Can you work these out from the model? Positions are in its coordinate system, mm. A direction names the side the tool comes from. Round coordinates to 2 decimals unless told otherwise and drop trailing zeros. Write each loop counter-clockwise with the first axis right and the second up, starting at its lowest first coordinate (ties: lowest second). Pieces come first, ordered by that corner, then holes.
Q1. We'd pull the mould along Y, two halves only. Please class faces 1 (the flat face through (9.75, 0, 1)), 2 (the flat face through (-11.5, 0, 1)), 3 (the flat face through (-10, 42, 1)), 4 (the flat face through (-7.5, -43, 1)): +Y half, -Y half, draft (parallel to the pull), parting line (faces both ways), or undercut.
Q2. If we section it at C-C (z = 0.9): Give the number of separate pieces and of enclosed holes in the cut face, plus the area to 3 significant figures.
Q3. If we section it at A-A (x = 0): Please give me the cut outline in (y, z), plus the area to 3 significant figures.
Q4. For faces 5 (the flat face through (7.5, 43, 1)), 6 (the flat face through (5.25, 0, 1)), 7 (the flat face through (-7.5, 43, 1)), 8 (the flat face through (2, -42, 1)), which set-ups out of +Z, -Z, +X, -X, +Y, -Y let a thin tool reach every point of the face, with its end or its side?
Q5. If we section it at D-D (x = -5.5): Please give me the cut outline in (y, z).
Q6. If we section it at B-B (y = -27): Please give me the cut outline in (x, z), plus the area to 3 significant figures.
Q7. Please list where these lines run through material, in increasing order: line 1 along Y through (x, z) = (-8.65, 0.95); line 2 along Y through (x, z) = (0.5, 1.8); line 3 along Y through (x, z) = (-10.75, 1.6).
Q8. I'm going to push flat-ended pins straight in: pin 1 Ø0.9 at (y, z) = (43.5, 1.5) entering from -X; pin 2 Ø0.9 at (y, z) = (-29, 1) entering from -X; pin 3 Ø1.6 at (x, z) = (-11, 1) entering from -Y; pin 4 Ø1.2 at (x, y) = (-8.65, -21.175) entering from -Z. Where does each tip first touch, or does it pass through?
from build123d import *

# Parameters (mm, degrees)
CROQUIS2_W              = 25
CROQUIS2_H              = 90
SALIENTE_EXTRUIR1_DEPTH = 3
CROQUIS3_W              = 10
CROQUIS3_H              = 3
CROQUIS3_W_2            = 5
CORTAR_EXTRUIR1_DEPTH   = 47.800106837
CROQUIS5_R              = 8.5
CROQUIS5_R_2            = 0.975
CORTAR_EXTRUIR2_DEPTH   = 47.800106837
CROQUIS6_W              = 2
CROQUIS6_H              = 11
CORTAR_EXTRUIR3_DEPTH   = 10
CROQUIS7_W              = 3
CROQUIS7_H              = 25
SALIENTE_EXTRUIR2_DEPTH = 3
CHAFL_N1_SIZE           = 3


with BuildPart() as part:
    # Croquis2 → Saliente-Extruir1 (new body)
    with BuildSketch(Plane.XY):
        Rectangle(CROQUIS2_W, CROQUIS2_H)
    extrude(amount=SALIENTE_EXTRUIR1_DEPTH)

    # Croquis3 → Cortar-Extruir1 (cut, through all)
    with BuildSketch(Plane.XY):
        with Locations((2.5, 43.5)):
            Rectangle(CROQUIS3_W, CROQUIS3_H)
        with Locations((-10, 43.5)):
            Rectangle(CROQUIS3_W_2, CROQUIS3_H)
    cortar_extruir1 = extrude(amount=CORTAR_EXTRUIR1_DEPTH, mode=Mode.SUBTRACT)

    # Simetría2: Cortar-Extruir1 across plane
    add(cortar_extruir1.mirror(Plane.ZX), mode=Mode.SUBTRACT)

    # Croquis5 → Cortar-Extruir2 (cut, through all)
    with BuildSketch(Plane.XY):
        with Locations((0, 12.95)):
            Circle(CROQUIS5_R)
        with Locations((0, -12.95)):
            Circle(CROQUIS5_R)
        with Locations((-8.65, 21.175)):
            Circle(CROQUIS5_R_2)
        with Locations((8.65, 21.175)):
            Circle(CROQUIS5_R_2)
        with Locations((8.65, -21.175)):
            Circle(CROQUIS5_R_2)
        with Locations((-8.65, -21.175)):
            Circle(CROQUIS5_R_2)
        with BuildLine():
            Line((9.75, -3.25), (9.75, 3.25))
            ThreePointArc((9.75, 3.25), (7.5, 5.5), (5.25, 3.25))
            Line((5.25, 3.25), (5.25, -3.25))
            ThreePointArc((5.25, -3.25), (7.5, -5.5), (9.75, -3.25))
        make_face()
    extrude(amount=CORTAR_EXTRUIR2_DEPTH, mode=Mode.SUBTRACT)

    # Croquis6 → Cortar-Extruir3 (cut)
    with BuildSketch(Plane.XY):
        with Locations((-10.5, 0)):
            Rectangle(CROQUIS6_W, CROQUIS6_H)
    extrude(amount=CORTAR_EXTRUIR3_DEPTH, mode=Mode.SUBTRACT)

    # Croquis7 → Saliente-Extruir2 (add)
    with BuildSketch(Plane.XY):
        with Locations((-14, 0)):
            Rectangle(CROQUIS7_W, CROQUIS7_H)
    extrude(amount=SALIENTE_EXTRUIR2_DEPTH)

    # Chaflán1
    chafl_n1_edges = [part.edges().sort_by_distance(p)[0] for p in [
        (-12.5, -12.5, 1.5),
        (-12.5, 12.5, 1.5),
    ]]
    chamfer(chafl_n1_edges, length=CHAFL_N1_SIZE - 0.0001)  # a hair under: the kernel refuses the full size


solid = part.part
A:
1. face 1: undercut
1. face 2: undercut
1. face 3: +Y half
1. face 4: draft
2. separate pieces: 1
2. enclosed holes: 8
2. area: 1,710 mm2
3. outline: (-42, 0) - (-21.45, 0) - (-21.45, 3) - (-42, 3) - close; (-4.45, 0) - (4.45, 0) - (4.45, 3) - (-4.45, 3) - close; (21.45, 0) - (42, 0) - (42, 3) - (21.45, 3) - close
3. area: 150 mm2
4. face 5: +Z, -Z, +Y
4. face 6: +Z, -Z
4. face 7: +Z, -Z, -X, +Y
4. face 8: +Z, -Z, -Y
5. outline: (-45, 0) - (-19.43, 0) - (-19.43, 3) - (-45, 3) - close; (-6.47, 0) - (6.47, 0) - (6.47, 3) - (-6.47, 3) - close; (19.43, 0) - (45, 0) - (45, 3) - (19.43, 3) - close
6. outline: (-12.5, 0) - (12.5, 0) - (12.5, 3) - (-12.5, 3) - close
6. area: 75.0 mm2
7. line 1: y = -42 to -22.15, -20.2 to 20.2, 22.15 to 42
7. line 2: y = -42 to -21.44, -4.46 to 4.46, 21.44 to 42
7. line 3: y = -42 to -5.5, 5.5 to 42
8. pin 1: stops at x = -7.5
8. pin 2: stops at x = -12.5
8. pin 3: stops at y = -42
8. pin 4: passes through
